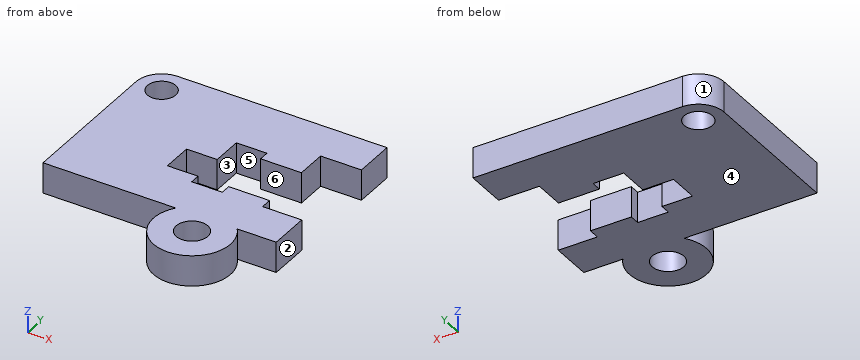
from build123d import *

# Parameters (mm, degrees)
F0_R     = 3.929234
F0_R_2   = 3.528575
F1_DEPTH = 7.62


with BuildPart() as f1:
    # F0 (on Top) → F1 (new body)
    with BuildSketch(Plane.XY):
        with BuildLine():
            Line((0.427139, 33.241566), (-51.642861, 33.241566))
            ThreePointArc((-51.642861, 33.241566), (-56.132989, 31.381694), (-57.992861, 26.891566))
            Line((-57.992861, 26.891566), (-57.992861, -10.16))
            Line((-57.992861, -10.16), (-24.972861, -10.16))
            ThreePointArc((-24.972861, -10.16), (-17.335705, -25.499214), (-9.69855, -10.16))
            Line((-9.69855, -10.16), (0, -10.16))
            Line((0, -10.16), (0, 0))
            Line((0, 0), (-9.732861, 0))
            Line((-9.732861, 0), (-9.732861, 2.761566))
            Line((-9.732861, 2.761566), (-19.892861, 2.761566))
            Line((-19.892861, 2.761566), (-19.892861, 0.221566))
            Line((-19.892861, 0.221566), (-27.512861, 0.221566))
            Line((-27.512861, 0.221566), (-27.512861, 2.761566))
            Line((-27.512861, 2.761566), (-35.132861, 2.761566))
            Line((-35.132861, 2.761566), (-35.132861, 10.381566))
            Line((-35.132861, 10.381566), (-27.512861, 10.381566))
            Line((-27.512861, 10.381566), (-27.512861, 18.001566))
            Line((-27.512861, 18.001566), (-19.892861, 18.001566))
            Line((-19.892861, 18.001566), (-19.892861, 15.461566))
            Line((-19.892861, 15.461566), (-9.732861, 15.461566))
            Line((-9.732861, 15.461566), (-9.732861, 23.081566))
            Line((-9.732861, 23.081566), (0.427139, 23.081566))
            Line((0.427139, 23.081566), (0.427139, 33.241566))
        make_face()
        with Locations((-17.335705, -15.928397)):
            Circle(F0_R, mode=Mode.SUBTRACT)
        with Locations((-51.642861, 26.891566)):
            Circle(F0_R_2, mode=Mode.SUBTRACT)
    extrude(amount=F1_DEPTH)


solid = f1.part
The model under review builds one solid part; all positions refer to its coordinate system, in mm. Face numbers are marked on the shaded views. A direction names the side the tool comes from. Coordinates: 2 decimals unless noted, no trailing zeros. Loops run counter-clockwise (first coordinate to the right, second up) from the corner with the lowest first, then second, coordinate; pieces in that order, holes last. Notation, with made-up numbers: (5.5, 78) -> (59.5, 78) arc R19 cw to (59.5, 102) -> close; hole circle Ø5 at (-11, 80). An arc over 180 degrees is marked (long way). Use a Markdown table: item, result. Add a question column.
1. Add section D-D on y = 8.5. Write out the cut boundary in (x, z).
2. Clearance check with flat-ended pins moving along their axes: pin 1 Ø1.5 at (x, z) = (-28.5, 2) entering from -Y; pin 2 Ø4 at (y, z) = (14.5, 4) entering from +X; pin 3 Ø2.5 at (y, z) = (-5.5, 2) entering from +X; pin 4 Ø10 at (x, y) = (-23.5, 19.5) entering from -Z. State where each tip first meets the part, or that it passes through.
3. Add section A-A on y = -19. Write out the cut boundary in (x, z), plus the area to 3 significant figures.
4. To check wall thickness, follow line 1 (Y direction, x = -35, z = 4.75); line 2 (Y direction, x = -2.5, z = 3); line 3 (X direction, y = 17.5, z = 1.5). State the ranges of each line that lie inside material, in increasing order.
5. Machinability: for the marked faces 4, 5 and 6, which of the approach directions +Z, -Z, +X, -X, +Y, -Y give a long, thin tool a straight path to every point of the face, cutting with its end or side? Answer none if there is none.
6. Add section B-B on x = -29. Write out the cut boundary in (y, z).
7. Draft analysis for pull direction Y (two halves, no side actions). For the marked faces 1, 2 and 3, state which applies: pulls with the +Y half, pulls with the -Y half, needs draft (parallel to the pull), parting line crosses it, or undercut.
8. Add section C-C on z = 4. Write out the cut boundary in (x, y), plus the area to 3 significant figures.
Returned:
| question | item | result |
|---|---|---|
| 1 | outline | (-57.99, 0) -> (-35.13, 0) -> (-35.13, 7.62) -> (-57.99, 7.62) -> close |
| 2 | pin 1 | stops at y = -10.16 |
| 2 | pin 2 | stops at x = -9.73 |
| 2 | pin 3 | stops at x = 0 |
| 2 | pin 4 | stops at z = 0 |
| 3 | outline | (-26.4, 0) -> (-19.79, 0) -> (-19.79, 7.62) -> (-26.4, 7.62) -> close; (-14.89, 0) -> (-8.27, 0) -> (-8.27, 7.62) -> (-14.89, 7.62) -> close |
| 3 | area | 101 mm² |
| 4 | line 1 | y = -10.16 to 2.76, 10.38 to 33.24 |
| 4 | line 2 | y = -10.16 to 0, 23.08 to 33.24 |
| 4 | line 3 | x = -57.99 to -27.51, -19.89 to -9.73 |
| 5 | face 4 | -Z, +X, -X, +Y, -Y |
| 5 | face 5 | +Z, -Z |
| 5 | face 6 | +Z, -Z, +X |
| 6 | outline | (-10.16, 0) -> (2.76, 0) -> (2.76, 7.62) -> (-10.16, 7.62) -> close; (10.38, 0) -> (33.24, 0) -> (33.24, 7.62) -> (10.38, 7.62) -> close |
| 7 | face 1 | pulls with the +Y half |
| 7 | face 2 | needs draft |
| 7 | face 3 | undercut |
| 8 | outline | (-57.99, -10.16) -> (-24.97, -10.16) arc R9.57 ccw (long way) to (-9.7, -10.16) -> (0, -10.16) -> (0, 0) -> (-9.73, 0) -> (-9.73, 2.76) -> (-19.89, 2.76) -> (-19.89, 0.22) -> (-27.51, 0.22) -> (-27.51, 2.76) -> (-35.13, 2.76) -> (-35.13, 10.38) -> (-27.51, 10.38) -> (-27.51, 18) -> (-19.89, 18) -> (-19.89, 15.46) -> (-9.73, 15.46) -> (-9.73, 23.08) -> (0.43, 23.08) -> (0.43, 33.24) -> (-51.64, 33.24) arc R6.35 ccw to (-57.99, 26.89) -> close; hole circle Ø7.06 at (-51.64, 26.89); hole circle Ø7.86 at (-17.34, -15.93) |
| 8 | area | 2,130 mm² |
